```python
from build123d import *

# Parameters (mm, degrees)
F1_DEPTH       = 460
F3_D           = 6.5
F3_DEPTH       = 15
F3_CBORE_D     = 11
F3_CBORE_DEPTH = 5
F5_D           = 6.5
F5_DEPTH       = 15
F5_CBORE_D     = 12
F5_CBORE_DEPTH = 2
F6_W           = 30
F6_H           = 15
F7_DEPTH       = 5


with BuildPart() as f1:
    # F0 (on Front) → F1 (new body)
    with BuildSketch(Plane.XZ):
        Polygon((0, 15), (0, 0), (30, 0), (30, 10), (20, 10), (20, 15), align=None)
    extrude(amount=-F1_DEPTH)

    # F3
    with Locations(Plane(origin=(0, 0, 0), x_dir=(1, 0, 0), z_dir=(0, 0, -1))):
        with Locations((10, -440), (10, -230), (10, -20)):
            CounterBoreHole(F3_D / 2, F3_CBORE_D / 2, F3_CBORE_DEPTH, depth=F3_DEPTH)

    # F5
    with Locations(Plane.XY.offset(15)):
        with Locations((10, 440), (10, 230), (10, 20)):
            CounterBoreHole(F5_D / 2, F5_CBORE_D / 2, F5_CBORE_DEPTH, depth=F5_DEPTH)

    # F6 (on face) → F7 (join)
    with BuildSketch(Plane(origin=(0, 460, 0), x_dir=(-1, 0, 0), z_dir=(0, 1, 0))):
        with Locations((-15, 7.5)):
            Rectangle(F6_W, F6_H)
    extrude(amount=F7_DEPTH)


solid = f1.part
```
Check sheet for the modelled part. Datum: model origin and axes. Units: mm. A direction names the side the tool comes from. Round coordinates to 2 decimals unless told otherwise and drop trailing zeros. Order: outer loops, then holes, each group sorted by start corner. A loop starts at its lowest first (then second) coordinate and runs counter-clockwise, first axis right, second up.
1) Mould release check, pull along X, two halves, no side actions. Record for faces 1 (the flat face through (25, 227, 10)), 2 (the flat face through (30, 229, 6)), 3 (the cylindrical face through (9.22, 445.95, 14.01)): +X half, -X half, draft (parallel to the pull), parting line (faces both ways), or undercut.
2) Section check A-A (z = 2.5). Record the boundary of the cut face in (x, y), and give its area (3 significant figures).
3) Scan lines: line 1 (Y direction, x = 9.75, z = 9); line 2 (Y direction, x = 10, z = 3.5); line 3 (X direction, y = 230, z = 2.2). Record each from-to range of solid material in increasing order.
4) Go/stop test with flat-tipped pins: pin 1 Ø3 at (x, y) = (26.5, 160.5) entering from +Z; pin 2 Ø4 at (x, y) = (10, 440) entering from -Z; pin 3 Ø10 at (x, y) = (10, 230) entering from -Z; pin 4 Ø6 at (x, y) = (12, 438.5) entering from +Z. Record where each tip stops, or that it passes through.
5) Section check C-C (x = 25). Record the boundary of the cut face in (y, z), and give its area (4 significant figures).
6) Tool access check on faces 4 (the flat face through (15, 465, 8)), 5 (the cylindrical face through (8.81, 235.37, 2.46)), 6 (the flat face through (13, 437, 13)). Record the directions out of +Z, -Z, +X, -X, +Y, -Y that give a thin tool (end or side, any length) a straight path to the whole face; none if there is none.
7) Section check B-B (y = 187). Record the boundary of the cut face in (x, z), and give its area (3 significant figures).
Result:
1. face 1: draft
1. face 2: +X half
1. face 3: undercut
2. outline: (0, 0) - (30, 0) - (30, 465) - (0, 465) - close; hole circle Ø11 at (10, 20); hole circle Ø11 at (10, 230); hole circle Ø11 at (10, 440)
2. area: 13,700 mm2
3. line 1: y = 0 to 16.76, 23.24 to 226.76, 233.24 to 436.76, 443.24 to 465
3. line 2: y = 0 to 14.5, 25.5 to 224.5, 235.5 to 434.5, 445.5 to 465
3. line 3: x = 0 to 4.5, 15.5 to 30
4. pin 1: stops at z = 10
4. pin 2: passes through
4. pin 3: stops at z = 5
4. pin 4: stops at z = 13
5. outline: (0, 0) - (465, 0) - (465, 15) - (460, 15) - (460, 10) - (0, 10) - close
5. area: 4,675 mm2
6. face 4: +Z, -Z, +X, -X, +Y
6. face 5: -Z
6. face 6: +Z
7. outline: (0, 0) - (30, 0) - (30, 10) - (20, 10) - (20, 15) - (0, 15) - close
7. area: 400 mm2
